Can you work these out from the model? Positions are in its coordinate system, mm. Face numbers are marked on the shaded views. A direction names the side the tool comes from. Coordinates: 2 decimals unless noted, no trailing zeros. Write each loop counter-clockwise with the first axis right and the second up, starting at its lowest first coordinate (ties: lowest second). Pieces come first, ordered by that corner, then holes.
```python
from build123d import *

# Parameters (mm, degrees)
F0_W        = 110
F0_H        = 69
F0_R        = 5.25
F0_W_2      = 5
F0_H_2      = 44
F1_DEPTH    = 12
F2_T1_DEPTH = 12
F2_T3_DEPTH = 37


# Not quite as in the source:
# - a fillet or chamfer that OpenCascade refuses, or shapes differently, is made with other operations: its cross-section is extruded or revolved along the edge and cut away or added


with BuildPart() as f1:
    # F0 (on Top) → F1 (new body)
    with BuildSketch(Plane.XY):
        Rectangle(F0_W, F0_H)
        with Locations((-43, -23)):
            Circle(F0_R, mode=Mode.SUBTRACT)
        with Locations((43, -23)):
            Circle(F0_R, mode=Mode.SUBTRACT)
        with Locations((-43, 23)):
            Circle(F0_R, mode=Mode.SUBTRACT)
        Polygon((30.5, 22), (30.5, -22), (2.5, -22), (-2.5, -22), (-30.5, -22), (-30.5, 22), (-2.5, 22), (2.5, 22), align=None, mode=Mode.SUBTRACT)
        with Locations((43, 23)):
            Circle(F0_R, mode=Mode.SUBTRACT)
        Rectangle(F0_W_2, F0_H_2)
    extrude(amount=F1_DEPTH)

    # F2: fillet of radius 5 on 12 edges, made by hand

    # F2_s2 → F2_t1 (join)
    with BuildSketch(Plane.XY):
        with BuildLine():
            add(Edge.make_bspline(
                [(-30.5, 17), (-30.5, 22), (-25.5, 22)],
                knots=[0, 0, 0, 1, 1, 1], degree=2, weights=[1, 1, 1]))
            Line((-25.5, 22), (-30.5, 22))
            Line((-30.5, 22), (-30.5, 17))
        make_face()
        with BuildLine():
            add(Edge.make_bspline(
                [(2.5, 17), (2.5, 22), (7.5, 22)],
                knots=[0, 0, 0, 1, 1, 1], degree=2, weights=[1, 1, 1]))
            Line((7.5, 22), (2.5, 22))
            Line((2.5, 22), (2.5, 17))
        make_face()
        with BuildLine():
            add(Edge.make_bspline(
                [(30.5, -17), (30.5, -22), (25.5, -22)],
                knots=[0, 0, 0, 1, 1, 1], degree=2, weights=[1, 1, 1]))
            Line((25.5, -22), (30.5, -22))
            Line((30.5, -22), (30.5, -17))
        make_face()
        with BuildLine():
            add(Edge.make_bspline(
                [(-7.5, -22), (-2.5, -22), (-2.5, -17)],
                knots=[0, 0, 0, 1, 1, 1], degree=2, weights=[1, 1, 1]))
            Line((-2.5, -17), (-2.5, -22))
            Line((-2.5, -22), (-7.5, -22))
        make_face()
        with BuildLine():
            add(Edge.make_bspline(
                [(30.5, 17), (30.5, 22), (25.5, 22)],
                knots=[0, 0, 0, 1, 1, 1], degree=2, weights=[1, 1, 1]))
            Line((25.5, 22), (30.5, 22))
            Line((30.5, 22), (30.5, 17))
        make_face()
        with BuildLine():
            add(Edge.make_bspline(
                [(-7.5, 22), (-2.5, 22), (-2.5, 17)],
                knots=[0, 0, 0, 1, 1, 1], degree=2, weights=[1, 1, 1]))
            Line((-2.5, 17), (-2.5, 22))
            Line((-2.5, 22), (-7.5, 22))
        make_face()
        with BuildLine():
            add(Edge.make_bspline(
                [(-25.5, -22), (-30.5, -22), (-30.5, -17)],
                knots=[0, 0, 0, 1, 1, 1], degree=2, weights=[1, 1, 1]))
            Line((-30.5, -17), (-30.5, -22))
            Line((-30.5, -22), (-25.5, -22))
        make_face()
        with BuildLine():
            add(Edge.make_bspline(
                [(7.5, -22), (2.5, -22), (2.5, -17)],
                knots=[0, 0, 0, 1, 1, 1], degree=2, weights=[1, 1, 1]))
            Line((2.5, -17), (2.5, -22))
            Line((2.5, -22), (7.5, -22))
        make_face()
    extrude(amount=F2_T1_DEPTH)

    # F2_s4 → F2_t3 (cut)
    with BuildSketch(Plane.XY.offset(-12.5)):
        with BuildLine():
            add(Edge.make_bspline(
                [(55, -29.5), (55, -34.5), (50, -34.5)],
                knots=[0, 0, 0, 1, 1, 1], degree=2, weights=[1, 1, 1]))
            Line((50, -34.5), (55, -34.5))
            Line((55, -34.5), (55, -29.5))
        make_face()
        with BuildLine():
            add(Edge.make_bspline(
                [(50, 34.5), (55, 34.5), (55, 29.5)],
                knots=[0, 0, 0, 1, 1, 1], degree=2, weights=[1, 1, 1]))
            Line((55, 29.5), (55, 34.5))
            Line((55, 34.5), (50, 34.5))
        make_face()
        with BuildLine():
            add(Edge.make_bspline(
                [(-55, -29.5), (-55, -34.5), (-50, -34.5)],
                knots=[0, 0, 0, 1, 1, 1], degree=2, weights=[1, 1, 1]))
            Line((-50, -34.5), (-55, -34.5))
            Line((-55, -34.5), (-55, -29.5))
        make_face()
        with BuildLine():
            add(Edge.make_bspline(
                [(-50, 34.5), (-55, 34.5), (-55, 29.5)],
                knots=[0, 0, 0, 1, 1, 1], degree=2, weights=[1, 1, 1]))
            Line((-55, 29.5), (-55, 34.5))
            Line((-55, 34.5), (-50, 34.5))
        make_face()
    extrude(amount=F2_T3_DEPTH, mode=Mode.SUBTRACT)


solid = f1.part
```
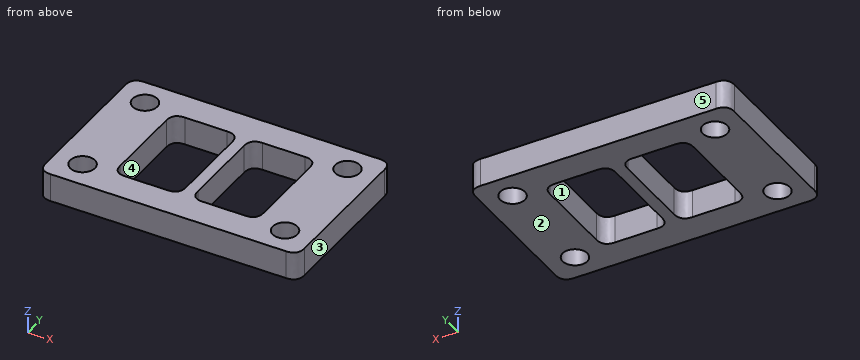
1. If we section it at D-D, the plane z = 9.75: Count the separate pieces of the cut face and the enclosed holes in it, plus the area to 3 significant figures.
2. If I drill on L1, parallel to Y at x = 43, z = 6; L2, parallel to X at y = 3.5, z = 7.5; L3, parallel to Y at x = -20.5, z = 3.5, over which ranges is the centre line in solid material (lowest first)?
3. If we section it at A-A, the plane x = 24: List the corners of the cut face in (y, z) for me.
4. If we section it at B-B, the plane y = -5: List the corners of the cut face in (x, z) for me.
5. If we section it at C-C, the plane x = 43: List the corners of the cut face in (y, z) for me.
6. Which directions (+Z, -Z, +X, -X, +Y, -Y) give clear straight access to the entire face, cutting with the end or side of a thin tool? Please do the marked faces 1 and 2.
7. We'd pull the mould along Y, two halves only. Please class the marked faces 3, 4 and 5: released by +Y, released by -Y, zero draft, split by the parting line, or undercut.
Answers:
1. separate pieces: 1
1. enclosed holes: 6
1. area: 4,800 mm2
2. L1: y = -34.5 to -28.25, -17.75 to 17.75, 28.25 to 34.5
2. L2: x = -55 to -30.5, -2.5 to 2.5, 30.5 to 55
2. L3: y = -34.5 to -22, 22 to 34.5
3. outline: (-34.5, 0) - (-22, 0) - (-22, 12) - (-34.5, 12) - close; (22, 0) - (34.5, 0) - (34.5, 12) - (22, 12) - close
4. outline: (-55, 0) - (-30.5, 0) - (-30.5, 12) - (-55, 12) - close; (-2.5, 0) - (2.5, 0) - (2.5, 12) - (-2.5, 12) - close; (30.5, 0) - (55, 0) - (55, 12) - (30.5, 12) - close
5. outline: (-34.5, 0) - (-28.25, 0) - (-28.25, 12) - (-34.5, 12) - close; (-17.75, 0) - (17.75, 0) - (17.75, 12) - (-17.75, 12) - close; (28.25, 0) - (34.5, 0) - (34.5, 12) - (28.25, 12) - close
6. face 1: +Z, -Z
6. face 2: -Z, +X, -X, +Y, -Y
7. face 3: zero draft
7. face 4: undercut
7. face 5: released by +Y
